Verification items for this drawing (mm, ordinates from the low corner). A direction names the side the tool comes from. Round coordinates to 2 decimals unless told otherwise and drop trailing zeros. Loops run counter-clockwise (first coordinate to the right, second up) from the corner with the lowest first, then second, coordinate; pieces in that order, holes last. Notation, with made-up numbers: (-33, -10.75) -> (-23, -10.75) arc R16 cw to (-23, 3.25) -> close; hole circle Ø2 at (42, 71.5). An arc over 180 degrees is marked (long way). One line per question, with ' | ' between items.
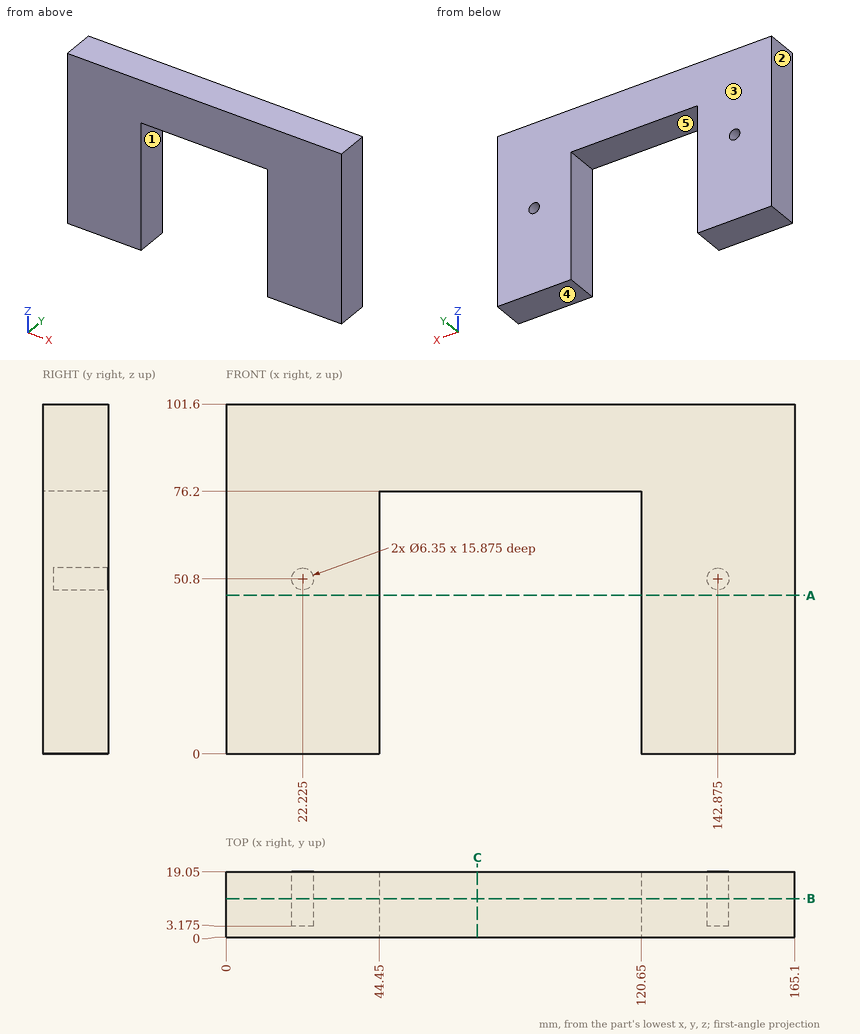
(1) Sectioned sample at C-C, the plane x = 73. Record the cut outline in (y, z), and give its area (3 significant figures).
Answer:
outline: (0, 76.2) -> (19.05, 76.2) -> (19.05, 101.6) -> (0, 101.6) -> close | area: 484 mm2
(2) Scan lines: probe 1 along X at (y, z) = (13.75, 50.8); probe 2 along X at (y, z) = (16.75, 25); probe 3 along Z at (x, y) = (105, 10.5). Record each from-to range of solid material in increasing order.
Answer:
probe 1: x = 0 to 19.05, 25.4 to 44.45, 120.65 to 139.7, 146.05 to 165.1 | probe 2: x = 0 to 44.45, 120.65 to 165.1 | probe 3: z = 76.2 to 101.6
(3) Sectioned sample at A-A, the plane z = 46. Record the cut outline in (x, y), and give its area (3 significant figures).
Answer:
outline: (0, 0) -> (44.45, 0) -> (44.45, 19.05) -> (0, 19.05) -> close; (120.65, 0) -> (165.1, 0) -> (165.1, 19.05) -> (120.65, 19.05) -> close | area: 1,690 mm2
(4) Set-up check for the marked faces 4 and 5: record each of +Z, -Z, +X, -X, +Y, -Y from which the full face is reachable in a straight line by a thin tool's end or side.
Answer:
face 4: -Z, +X, -X, +Y, -Y | face 5: -Z, +Y, -Y
(5) Sectioned sample at B-B, the plane y = 11.25. Record the cut outline in (x, z) (3 decimals), and give its area (3 significant figures).
Answer:
outline: (0, 0) -> (44.45, 0) -> (44.45, 76.2) -> (120.65, 76.2) -> (120.65, 0) -> (165.1, 0) -> (165.1, 101.6) -> (0, 101.6) -> close; hole circle Ø6.35 at (22.225, 50.8); hole circle Ø6.35 at (142.875, 50.8) | area: 10,900 mm2
(6) Go/stop test with a flat-tipped pin: pin 1 (5.5 mm diameter, centred on x = 22.225, z = 50.8, fed in from +Y) (3 decimals). Record where the tip stops, or that it passes through.
Answer:
pin 1: stops at y = 3.175
(7) Mould release check, pull along X, two halves, no side actions. Record for the marked faces 1, 2 and 3: +X half, -X half, draft (parallel to the pull), parting line (faces both ways), or undercut.
Answer:
face 1: undercut | face 2: -X half | face 3: draft
